Geometry: final body of the model. Coordinates: model frame, mm. A direction names the side the tool comes from. Round coordinates to 2 decimals unless told otherwise and drop trailing zeros. Loops run counter-clockwise (first coordinate to the right, second up) from the corner with the lowest first, then second, coordinate; pieces in that order, holes last. Notation, with made-up numbers: (80.25, 89) - (99.25, 89) arc R34 ccw to (99.25, 121) - close; hole circle Ø6 at (38, -0.5). An arc over 180 degrees is marked (long way). Answer as CSV lines item,"result".
from build123d import *

# Parameters (mm, degrees)
SKETCH1_W           = 100
SKETCH1_H           = 80
BOSS_EXTRUDE1_DEPTH = 60
CUT_EXTRUDE1_DEPTH  = 60


with BuildPart() as part:
    # Sketch1 → Boss-Extrude1 (new body)
    with BuildSketch(Plane(origin=(0, 0, 0), x_dir=(1, 0, 0), z_dir=(0, 1, 0))):
        Rectangle(SKETCH1_W, SKETCH1_H)
    extrude(amount=BOSS_EXTRUDE1_DEPTH)

    # Sketch2 → Cut-Extrude1 (cut)
    with BuildSketch(Plane.XY.offset(40)):
        Polygon((-50, 60), (25, 60), (25, 45), (0, 45), (0, 30), (-25, 30), (-25, 15), (-50, 15), align=None)
    extrude(amount=-CUT_EXTRUDE1_DEPTH, mode=Mode.SUBTRACT)


solid = part.part
(1) Material intervals for line 1 along Z through (x, y) = (3, 57); line 2 along X through (y, z) = (53.5, 12); line 3 along Y through (x, z) = (20.5, 5.5), sorted ascending.
Findings below:
line 1,"-40 to -20"
line 2,"25 to 50"
line 3,"0 to 45"
(2) Pin query (flat end, axial travel): P1, Ø7.5, axis at x = -11, z = -1, coming from the +Y side; P2, Ø12, axis at y = 53.5, z = 25, coming from the -X side; P3, Ø20, axis at x = -39, z = 24, coming from the +Y side. Return the tip coordinate at first contact, or that it passes through.
Findings below:
P1,"y = 30"
P2,"x = 25"
P3,"y = 15"
(3) Access query for faces 1 (the face through (13, 45, 10)), 2 (the face through (-1, 30, -40)). Directions: +Z, -Z, +X, -X, +Y, -Y. A direction counts if a zero-diameter tool reaches every point of the face in a straight line with its end or side. Return the directions, or none.
Findings below:
face 1,"+Z, -X, +Y"
face 2,"-Z, +X, -X, +Y, -Y"
(4) Section C-C (y = 37). Output: boundary loops of the cut face in (x, z), and give its area (3 significant figures).
Findings below:
outline,"(-50, -40) - (50, -40) - (50, 40) - (0, 40) - (0, -20) - (-50, -20) - close"
area,"5,000 mm2"
(5) Section A-A (x = -17.5). Output: boundary loops of the cut face in (y, z).
Findings below:
outline,"(0, -40) - (60, -40) - (60, -20) - (30, -20) - (30, 40) - (0, 40) - close"
(6) Section B-B (z = 10.5). Output: boundary loops of the cut face in (x, y).
Findings below:
outline,"(-50, 0) - (50, 0) - (50, 60) - (25, 60) - (25, 45) - (0, 45) - (0, 30) - (-25, 30) - (-25, 15) - (-50, 15) - close"
